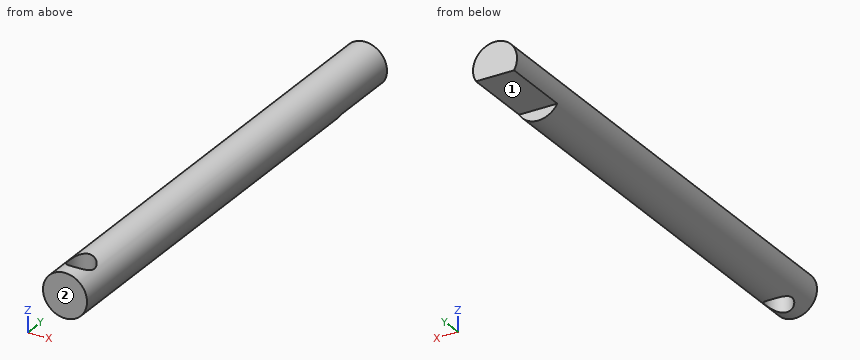
```python
from build123d import *

# Parameters (mm, degrees)
SKETCH1_R               = 3.96875
BOSS_EXTRUDE1_DEPTH     = 88.138
CUT_EXTRUDE1_DEPTH      = 12.7
CUT_EXTRUDE2_DEPTH      = 12.7
CUT_EXTRUDE2_DEPTH_BACK = 12.7
SKETCH3_R               = 2.38125


with BuildPart() as part:
    # Sketch1 → Boss-Extrude1 (new body)
    with BuildSketch(Plane(origin=(0, 0, 0), x_dir=(1, 0, 0), z_dir=(0, 1, 0))):
        with Locations(Location((0, 0, 0), (0, 0, 270))):
            Circle(SKETCH1_R)
    extrude(amount=BOSS_EXTRUDE1_DEPTH)

    # Sketch2 → Cut-Extrude1 (cut)
    with BuildSketch(Plane(origin=(0, 88.138, 0), x_dir=(1, 0, 0), z_dir=(0, 1, 0))):
        Polygon((3.437038321, 1.984375), (-3.437038321, 1.984375), (-4.719395918, 2.522465653), (-2.590204502, 6.353236507), (2.456720437, 4.728926773), align=None)
    extrude(amount=-CUT_EXTRUDE1_DEPTH, mode=Mode.SUBTRACT)

    # Sketch3 → Cut-Extrude2 (cut, two sides: drawn at the far end of the back side and taken through both)
    with BuildSketch(Plane(origin=(0, 0, -1.984375), x_dir=(-1, 0, 0), z_dir=(0, 0, -1)).offset(-CUT_EXTRUDE2_DEPTH_BACK)):
        with Locations(Location((0, 4.7625, 0), (0, 0, 180))):
            Circle(SKETCH3_R)
    extrude(amount=CUT_EXTRUDE2_DEPTH + CUT_EXTRUDE2_DEPTH_BACK, mode=Mode.SUBTRACT)


solid = part.part
```
Here's how the part is built. I have some questions about the finished solid (model axes, mm). Face numbers are marked on the shaded views. A direction names the side the tool comes from. Give positions to 0.01 mm unless a question says otherwise; leave off trailing zeros. Loops run counter-clockwise (first coordinate to the right, second up) from the corner with the lowest first, then second, coordinate; pieces in that order, holes last. Notation, with made-up numbers: (4.5, 80) -> (57.5, 80) arc R4 ccw to (57.5, 87) -> close; hole circle Ø9 at (36.25, -38.75). An arc over 180 degrees is marked (long way). Use one line per item in the form item = value. Start each with the question number.
1) For P1, Ø2, axis at x = 1.5, y = 83.5, coming from the -Z side; P2, Ø1.5, axis at y = 67, z = -3, coming from the -X side, each with a flat end and sliding along its axis, tell me the tip position at first contact or that it passes through.
2) Imagine slicing it at A-A (x = 0). Please give me the cut outline in (y, z), then the cut area to 3 significant figures.
3) Which directions (+Z, -Z, +X, -X, +Y, -Y) give clear straight access to the entire face, cutting with the end or side of a thin tool? Please do the marked faces 1 and 2.
4) Imagine slicing it at B-B (z = 0). Please give me the cut outline in (x, y), then the cut area to 3 significant figures.
5) Please list where these lines run through material, in increasing order: line 1 along Y through (x, z) = (0.25, 1.25); line 2 along Y through (x, z) = (0.75, -1.5); line 3 along Z through (x, y) = (0.25, 55).
6) Imagine slicing it at D-D (y = 79). Please give me the cut outline in (x, z), then the cut area to 3 significant figures.
7) Imagine slicing it at C-C (y = 34). Please give me the cut outline in (x, z).
Check values:
q1.P1 = -1.98
q1.P2 = -3.27
q2.outline = (0, -3.97) -> (2.38, -3.97) -> (2.38, 3.97) -> (0, 3.97) -> close; (7.14, -3.97) -> (75.44, -3.97) -> (75.44, -1.98) -> (88.14, -1.98) -> (88.14, 3.97) -> (7.14, 3.97) -> close
q2.area = 637 mm^2
q3.face_1 = -Z, +X, -X, +Y
q3.face_2 = +Z, -Z, +X, -X, -Y
q4.outline = (-3.97, 0) -> (3.97, 0) -> (3.97, 88.14) -> (-3.97, 88.14) -> close; hole circle Ø4.76 at (0, 4.76)
q4.area = 682 mm^2
q5.line_1 = 0 to 2.39, 7.13 to 88.14
q5.line_2 = 0 to 2.5, 7.02 to 88.14
q5.line_3 = -3.96 to 3.96
q6.outline = (-3.44, -1.98) -> (3.44, -1.98) arc R3.97 ccw (long way) to start
q6.area = 39.8 mm^2
q7.outline = circle Ø7.94 at (0, 0)
